Autodesk Fusion 360 part; units mm, degrees
sketch "Sketch1" plane through (0, 0, 0) normal (0, 0, 1) x (1, 0, 0)
  line L0 (44.45, 38.1) -> (-44.45, 38.1)
  line L1 (-44.45, 38.1) -> (-44.45, -38.1)
  line L2 (-44.45, -38.1) -> (44.45, -38.1)
  line L3 (44.45, -38.1) -> (44.45, 38.1)
  line L4 (44.45, 38.1) -> (-44.45, -38.1) construction
  line L5 (-44.45, 38.1) -> (44.45, -38.1) construction
  dimension "d1" = 88.9
  dimension "d2" = 76.2
extrude "Extrude1" add sketch "Sketch1" along normal blind 6.35
sketch "Sketch2" plane through (0, 0, 0) normal (0, 1, 0) x (1, 0, 0)
  line L0 (44.45, -6.35) -> (76.2, 25.4)
  line L1 (44.45, 0) -> (69.85, 25.4)
  line L2 (69.85, 25.4) -> (76.2, 25.4)
  line L3 (0, -50.8) -> (0, 63.5)
  line L4 (-69.85, 25.4) -> (-76.2, 25.4)
  line L5 (-44.45, 0) -> (-69.85, 25.4)
  line L6 (-44.45, -6.35) -> (-76.2, 25.4)
  line L7 (-44.45, -6.35) -> (-44.45, 0)
  line L8 (44.45, -6.35) -> (44.45, 0)
extrude "Extrude2" add sketch "Sketch2" along normal blind 38.1 and the other way blind 38.1
Can you work these out from the model? Positions are in its coordinate system, mm. A direction names the side the tool comes from. Coordinates: 2 decimals unless noted, no trailing zeros. Order: outer loops, then holes, each group sorted by start corner. A loop starts at its lowest first (then second) coordinate and runs counter-clockwise, first axis right, second up. Notation, with made-up numbers: (19, -17.5) - (50, -17.5) arc R24 ccw to (50, 6.5) - close; hole circle Ø3 at (38, -31). An arc over 180 degrees is marked (long way). Answer as a JSON object with one key per item and string values. Group by question number.
Q1. Imagine slicing it at C-C (x = -55.5). Please give me the cut outline in (y, z), and give its area (3 significant figures).
Q2. Imagine slicing it at B-B (y = 18). Please give me the cut outline in (x, z), and give its area (3 significant figures).
Q3. Imagine slicing it at A-A (z = -3.5). Please give me the cut outline in (x, y), and give its area (3 significant figures).
Q4. I need wall thicknesses on line 1 (Z direction, x = 42.5, y = -32); line 2 (X direction, y = -5.5, z = -17); line 3 (X direction, y = 24, z = -12). Which ranges of each line are inside material? Lowest first, please. Write a range as from..to.
Q5. Will these pins go through, and if not, where does the flat tip stop? P1, Ø3, axis at y = 16, z = 0.5, coming from the -X side; P2, Ø5, axis at y = -24.5, z = -10.5, coming from the +X side; P3, Ø5, axis at x = 58.5, y = 23.5, coming from the +Z side.
Q6. On a 3-axis mill with a long thin cutter (end or side, diameter ignored), from which of +Z, -Z, +X, -X, +Y, -Y can I reach the whole of each face in a straight line? I mean faces 4 (the face through (-56.97, -0.53, -12.52)), 5 (the face through (-73, -1, -25.4)). Say none if no direction works.
Q7. Imagine slicing it at D-D (z = 3). Please give me the cut outline in (x, y).
Q8. We'd pull the mould along X, two halves only. Please class faces 1 (the face through (-1, 1, 0)), 2 (the face through (-60.1, -0.5, -9.3)), 3 (the face through (73, -1, -25.4)): +X half, -X half, draft (parallel to the pull), parting line (faces both ways), or undercut.
Determined:
{
 "1": {"outline": "(-38.1, -11.05) - (38.1, -11.05) - (38.1, -4.7) - (-38.1, -4.7) - close", "area": "484 mm2"},
 "2": {"outline": "(-76.2, -25.4) - (-69.85, -25.4) - (-44.45, 0) - (44.45, 0) - (69.85, -25.4) - (76.2, -25.4) - (44.45, 6.35) - (-44.45, 6.35) - close", "area": "927 mm2"},
 "3": {"outline": "(-54.3, -38.1) - (-47.95, -38.1) - (-47.95, 38.1) - (-54.3, 38.1) - close; (47.95, -38.1) - (54.3, -38.1) - (54.3, 38.1) - (47.95, 38.1) - close", "area": "968 mm2"},
 "4": {"line 1": "z = 0..6.35", "line 2": "x = -67.8..-61.45, 61.45..67.8", "line 3": "x = -62.8..-56.45, 56.45..62.8"},
 "5": {"P1": "stops at x = -51.8", "P2": "stops at x = 63.8", "P3": "stops at z = -5.2"},
 "6": {"face 4": "-Z, +Y, -Y", "face 5": "-Z, +X, -X, +Y, -Y"},
 "7": {"outline": "(-47.8, -38.1) - (47.8, -38.1) - (47.8, 38.1) - (-47.8, 38.1) - close"},
 "8": {"face 1": "undercut", "face 2": "-X half", "face 3": "draft"}
}
